Verification items for the finished model (mm, model axes). Face numbers are marked on the shaded views. Give positions to 0.01 mm unless a question says otherwise; leave off trailing zeros. Write each loop counter-clockwise with the first axis right and the second up, starting at its lowest first coordinate (ties: lowest second). Pieces come first, ordered by that corner, then holes. Notation, with made-up numbers: (-31, -15.75) - (-4, -15.75) arc R32 ccw to (-4, 15.25) - close; hole circle Ø3 at (76.5, -8.5). An arc over 180 degrees is marked (long way). Answer as a JSON object with one key per item and string values. Group by question number.
Item 1: Draft check along Z on the marked faces 1, 2 and 3. Enter one of: +Z half, -Z half, draft (parallel to the pull), parting line (faces both ways), or undercut.
Item 2: Sectioned sample at D-D, the plane x = 24. Record the boundary of the cut face in (y, z).
Item 3: Sectioned sample at A-A, the plane z = 52. Record the boundary of the cut face in (x, y), and give its area (3 significant figures).
Item 4: Sectioned sample at C-C, the plane y = 16. Record the boundary of the cut face in (x, z).
Item 5: Go/stop test with flat-tipped pins: pin 1 (3 mm diameter, centred on y = 4.5, z = 18.5, fed in from +X); pin 2 (8 mm diameter, centred on y = 4, z = 38, fed in from -X); pin 3 (10 mm diameter, centred on x = 46.5, z = 15, fed in from +Y); pin 4 (1.5 mm diameter, centred on y = 6.5, z = 16.5, fed in from +X). Record where each tip stops, or that it passes through.
Item 6: Scan lines: line 1 along X through (y, z) = (1, 10); line 2 along Y through (x, z) = (16, 46); line 3 along Y through (x, z) = (13.5, 33). Record each from-to range of solid material in increasing order. Write a range as [from, to].
Item 7: Sectioned sample at B-B, the plane x = 6.5. Record the boundary of the cut face in (y, z), and give its area (3 significant figures).
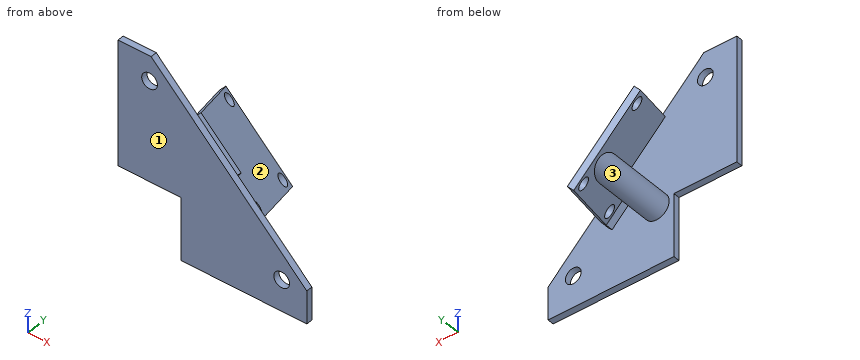
```python
from build123d import *

# Parameters (mm, degrees)
SKETCH_1_R      = 2.5
EXTRUDE_1_DEPTH = 2
SKETCH_2_R      = 2
EXTRUDE_3_DEPTH = 2
EXTRUDE_4_REACH = 91.774
SKETCH_4_R      = 4
EXTRUDE_5_REACH = 91.774


with BuildPart() as part:
    # Sketch 1 → Extrude 1 (new body)
    with BuildSketch(Plane(origin=(0, 0, 0), x_dir=(1, 0, 0), z_dir=(0, 1, 0))):
        Polygon((10.502525317, -60), (60, -10.502525317), (60, 0), (20, 0), (20, -20), (0, -20), (0, -60), align=None)
        with Locations(Location((10, -52, 0), (0, 0, 270))):
            Circle(SKETCH_1_R, mode=Mode.SUBTRACT)
        with Locations(Location((52, -10, 0), (0, 0, 270))):
            Circle(SKETCH_1_R, mode=Mode.SUBTRACT)
    extrude(amount=EXTRUDE_1_DEPTH)



with BuildPart() as body_2:
    # Sketch 2 → Extrude 3 (new body)
    with BuildSketch(Plane(origin=(23.112372436, 18.871173071, 23.112372436), x_dir=(-0.7071067811865475, 0, 0.7071067811865477), z_dir=(0.6123724356957955, 0.4999999999999981, 0.6123724356957954))):
        Polygon((-3, 16.786030205), (-15, 16.786030205), (-15, -13.213969795), (15, -13.213969795), (15, 9.786030205), (-3, 9.786030205), align=None)
        with Locations(Location((-12, -10.213969795, 0), (0, 0, 180))):
            Circle(SKETCH_2_R, mode=Mode.SUBTRACT)
        with Locations(Location((12, -10.213969795, 0), (0, 0, 180))):
            Circle(SKETCH_2_R, mode=Mode.SUBTRACT)
        with Locations(Location((-12, 13.786030205, 0), (0, 0, 180))):
            Circle(SKETCH_2_R, mode=Mode.SUBTRACT)
    extrude(amount=EXTRUDE_3_DEPTH)


with BuildPart() as part_1:
    add(part.part)

    add(body_2.part)  # Extrude 4 merges body 2
    # Extrude 4: up to this plane
    extrude_4_end = Plane(origin=(23.112372436, 18.871173071, 23.112372436), z_dir=(0.6123724356957954, 0.4999999999999981, 0.6123724356957952))
    # Sketch 4 → Extrude 4 (add, up to the surface)
    with BuildSketch(Plane(origin=(0, 2, 0), x_dir=(1, 0, 0), z_dir=(0, 1, 0)), mode=Mode.PRIVATE) as extrude_4_sk1:
        with Locations(Location((25.511596423, -18.440528611, 0), (0, 0, 315))):
            Circle(SKETCH_4_R)
    extrude_4_tool1 = split(extrude(extrude_4_sk1.sketch, amount=EXTRUDE_4_REACH, mode=Mode.PRIVATE), bisect_by=extrude_4_end, keep=Keep.BOTH, mode=Mode.PRIVATE)
    add(extrude_4_tool1.solids().sort_by_distance((25.511596, 2, 18.440529))[0])

    # Sketch 5 → Extrude 5 (add, up to next)
    with BuildSketch(Plane(origin=(0, 2, 0), x_dir=(1, 0, 0), z_dir=(0, 1, 0)), mode=Mode.PRIVATE) as extrude_5_sk1:
        Polygon((39.653732047, -18.440528611), (31.168450673, -26.925809986), (32.393195544, -28.150554857), (40.878476918, -19.665273483), align=None)
    extrude_5_tool1 = extrude(extrude_5_sk1.sketch, amount=EXTRUDE_5_REACH, mode=Mode.PRIVATE) - part_1.part
    add(extrude_5_tool1.solids().sort_by_distance((36.023464, 2, 23.295542))[0])


solid = part_1.part
```
Geometry check:
{
 "1": {"face 1": "draft", "face 2": "+Z half", "face 3": "undercut"},
 "2": {"outline": "(0, 0) - (2, 0) - (2, 14.74) - (28.04, 14.74) - (30.31, 12.88) - (31.31, 15.33) - (11.4, 31.59) - (10.4, 29.14) - (18.97, 22.14) - (2, 22.14) - (2, 46.5) - (0, 46.5) - close"},
 "3": {"outline": "(0, 0) - (7.5, 0) - (7.5, 2) - (0, 2) - close; (12.5, 0) - (18.5, 0) - (18.5, 2) - (12.5, 2) - close", "area": "27.0 mm^2"},
 "4": {"outline": "(13.68, 34.89) - (26.19, 22.38) arc R4 ccw (long way) to (29.45, 19.11) - (34.89, 13.68) - (36.52, 15.31) - (15.31, 36.52) - close"},
 "5": {"pin 1": "x = 40.88", "pin 2": "x = 0", "pin 3": "y = 2", "pin 4": "x = 29.33"},
 "6": {"line 1": "[20, 49.5], [54.5, 60]", "line 2": "[0, 2]", "line 3": "[0, 2], [18.53, 22.53]"},
 "7": {"outline": "(0, 20) - (2, 20) - (2, 60) - (0, 60) - close", "area": "80.0 mm^2"}
}
